```python
from build123d import *

# Parameters (mm, degrees)
F0_W     = 160
F0_H     = 110
F0_R     = 1
F1_DEPTH = 3
F2_W     = 160
F2_H     = 3
F3_DEPTH = 90
F4_R     = 6.5
F5_DEPTH = 110.001
F6_R     = 2


with BuildPart() as f1:
    # F0 (on Top) → F1 (new body)
    with BuildSketch(Plane.XY):
        Rectangle(F0_W, F0_H)
        with Locations((-65, 25)):
            Circle(F0_R, mode=Mode.SUBTRACT)
    extrude(amount=F1_DEPTH)

    # F2 (on face) → F3 (join)
    with BuildSketch(Plane(origin=(0, 0, 0), x_dir=(1, 0, 0), z_dir=(0, 0, -1))):
        with Locations((0, -53.5)):
            Rectangle(F2_W, F2_H)
    extrude(amount=F3_DEPTH)

    # F4 (on face) → F5 (cut, through all)
    with BuildSketch(Plane(origin=(0, 55, 0), x_dir=(-1, 0, 0), z_dir=(0, 1, 0))):
        with Locations((0, -78)):
            Circle(F4_R)
    extrude(amount=-F5_DEPTH, mode=Mode.SUBTRACT)

    # F6
    f6_edges = [f1.edges().sort_by_distance(p)[0] for p in [
        (0, 55, 3),
        (0, 52, 0),
    ]]
    fillet(f6_edges, radius=F6_R)


solid = f1.part
```
Geometry: final body of the model. Coordinates: model frame, mm. A direction names the side the tool comes from. Coordinates: 2 decimals unless noted, no trailing zeros. Order: outer loops, then holes, each group sorted by start corner. A loop starts at its lowest first (then second) coordinate and runs counter-clockwise, first axis right, second up. Notation, with made-up numbers: (-4, 78) -> (31, 78) arc R19 cw to (31, 95) -> close; hole circle Ø7 at (-4, 48). An arc over 180 degrees is marked (long way). Use CSV: the item, a comma, the result in double quotes.
1) Mould query, pull axis Z, two halves, no side actions, for faces 1 (the cylindrical face through (1.409, 53.521, -84.345)), 2 (the flat face through (-1, -2, 0)), 3 (the flat face through (-1, 55, -44)). Classes: +Z half, -Z half, draft (parallel to the pull), parting line (faces both ways), or undercut.
Findings:
face 1,"undercut"
face 2,"-Z half"
face 3,"draft"
2) Line query: line 1 (Y direction, x = 39, z = -76); line 2 (Z direction, x = -24, y = 14); line 3 (Z direction, x = 0, y = 54). Output: solid intervals per line, ascending.
Findings:
line 1,"y = 52 to 55"
line 2,"z = 0 to 3"
line 3,"z = -90 to -84.5, -71.5 to 2.73"
3) Pin query (flat end, axial travel): pin 1 Ø17 at (x, z) = (0, -78) entering from -Y; pin 2 Ø1 at (x, y) = (25.5, 44) entering from -Z. Return the tip coordinate at first contact, or that it passes through.
Findings:
pin 1,"stops at y = 52"
pin 2,"stops at z = 0"
4) Access query for faces 4 (the flat face through (-1, 52, -45)), 5 (the flat face through (-80, 25, 1)). Directions: +Z, -Z, +X, -X, +Y, -Y. A direction counts if a zero-diameter tool reaches every point of the face in a straight line with its end or side. Return the directions, or none.
Findings:
face 4,"-Z, +X, -X, -Y"
face 5,"+Z, -Z, -X, +Y, -Y"
5) Section D-D on y = 38. Output: boundary loops of the cut face in (x, z).
Findings:
outline,"(-80, 0) -> (80, 0) -> (80, 3) -> (-80, 3) -> close"
6) Section A-A on z = -73.5. Output: boundary loops of the cut face in (x, y), then the cut area to 3 significant figures.
Findings:
outline,"(-80, 52) -> (-4.69, 52) -> (-4.69, 55) -> (-80, 55) -> close; (4.69, 52) -> (80, 52) -> (80, 55) -> (4.69, 55) -> close"
area,"452 mm^2"
7) Section C-C on x = -18. Output: boundary loops of the cut face in (y, z), then the cut area to 3 significant figures.
Findings:
outline,"(-55, 0) -> (50, 0) arc R2 cw to (52, -2) -> (52, -90) -> (55, -90) -> (55, 1) arc R2 ccw to (53, 3) -> (-55, 3) -> close"
area,"600 mm^2"
8) Section B-B on x = 0. Output: boundary loops of the cut face in (y, z), then the cut area to 3 significant figures.
Findings:
outline,"(-55, 0) -> (50, 0) arc R2 cw to (52, -2) -> (52, -71.5) -> (55, -71.5) -> (55, 1) arc R2 ccw to (53, 3) -> (-55, 3) -> close; (52, -90) -> (55, -90) -> (55, -84.5) -> (52, -84.5) -> close"
area,"561 mm^2"
